```python
from build123d import *

# Parameters (mm, degrees)
SKETCH_1_R      = 1.4
SKETCH_1_W      = 12.8
SKETCH_1_H      = 6
SKETCH_1_W_2    = 15
SKETCH_1_W_3    = 6
SKETCH_1_H_2    = 10
EXTRUDE_1_DEPTH = 6


with BuildPart() as part:
    # Эскиз1 → Бобышка-Вытянуть1 (new body)
    with BuildSketch(Plane.XY):
        with BuildLine():
            Line((96.920798757, 2), (96.920798757, 25))
            Line((96.920798757, 25), (96.920798757, 33))
            ThreePointArc((96.920798757, 33), (98.385264851, 36.535533906), (101.920798757, 38))
            Line((101.920798757, 38), (149.389201243, 38))
            Line((149.389201243, 38), (149.389201243, 30))
            Line((149.389201243, 30), (149.389201243, 20.709265489))
            Line((149.389201243, 20.709265489), (143.389201243, 20.709265489))
            Line((143.389201243, 20.709265489), (143.389201243, 10.709265489))
            Line((143.389201243, 10.709265489), (149.389201243, 10.709265489))
            Line((149.389201243, 10.709265489), (149.389201243, -4.290734511))
            Line((149.389201243, -4.290734511), (143.389201243, -4.290734511))
            Line((143.389201243, -4.290734511), (143.389201243, -14.290734511))
            Line((143.389201243, -14.290734511), (149.389201243, -14.290734511))
            Line((149.389201243, -14.290734511), (149.389201243, -30))
            Line((149.389201243, -30), (-144.389201243, -30))
            Line((-144.389201243, -30), (-149.389201243, -25))
            Line((-149.389201243, -25), (-149.389201243, -13))
            Line((-149.389201243, -13), (81.920798757, -13))
            ThreePointArc((81.920798757, -13), (92.527400475, -8.606601718), (96.920798757, 2))
        make_face()
        with Locations((104.970798757, -19)):
            Circle(SKETCH_1_R, mode=Mode.SUBTRACT)
        with Locations((104.970798757, 25)):
            Circle(SKETCH_1_R, mode=Mode.SUBTRACT)
        with Locations((111.920798757, 3.209265489)):
            Circle(SKETCH_1_R, mode=Mode.SUBTRACT)
        with Locations((146.389201243, 3.209265489)):
            Circle(SKETCH_1_R, mode=Mode.SUBTRACT)
        with Locations((-128.98858016, -19)):
            Rectangle(SKETCH_1_W, SKETCH_1_H, mode=Mode.SUBTRACT)
        with Locations((-28.18858016, -19)):
            Rectangle(SKETCH_1_W, SKETCH_1_H, mode=Mode.SUBTRACT)
        with Locations((62.61141984, -19)):
            Rectangle(SKETCH_1_W, SKETCH_1_H, mode=Mode.SUBTRACT)
        with Locations((129.420798757, -19)):
            Rectangle(SKETCH_1_W_2, SKETCH_1_H, mode=Mode.SUBTRACT)
        with Locations((111.920798757, 15.709265489)):
            Rectangle(SKETCH_1_W_3, SKETCH_1_H_2, mode=Mode.SUBTRACT)
        with Locations((111.920798757, -9.290734511)):
            Rectangle(SKETCH_1_W_3, SKETCH_1_H_2, mode=Mode.SUBTRACT)
        with Locations((129.155798757, 33)):
            Rectangle(SKETCH_1_W_2, SKETCH_1_H, mode=Mode.SUBTRACT)
    extrude(amount=EXTRUDE_1_DEPTH)


solid = part.part
```
The model under review builds one solid part; all positions refer to its coordinate system, in mm. A direction names the side the tool comes from. Coordinates: 2 decimals unless noted, no trailing zeros. Write each loop counter-clockwise with the first axis right and the second up, starting at its lowest first coordinate (ties: lowest second). Pieces come first, ordered by that corner, then holes.
1) We need section B-B on x = -102. State the section outline as (y, z) points, then the cut area to 3 significant figures.
2) To check wall thickness, follow probe 1 along X at (y, z) = (-17, 2); probe 2 along Y at (x, z) = (135, 5.8); probe 3 along Y at (x, z) = (-128, 2.7). State the ranges of each line that lie inside material, in increasing order.
3) The part is to be moulded in two halves that separate along X. For faces 1 (the face through (-129, -22, 3)), 2 (the face through (149.389, 3, 3)), 3 (the face through (96.921, 17, 3)), say which applies: pulls with the +X half, pulls with the -X half, needs draft (parallel to the pull), parting line crosses it, or undercut.
4) We need section C-C on z = 2. Count the separate pieces of the cut face and the enclosed holes in it, then the cut area to 3 significant figures.
5) We need section A-A on y = -8.5. State the section outline as (x, z) points.
6) Clearance check with flat-ended pins moving along their axes: pin 1 Ø4.5 at (x, y) = (146.39, 3.21) entering from +Z; pin 2 Ø1.8 at (y, z) = (-7.5, 4) entering from +X; pin 3 Ø1.8 at (y, z) = (17, 4) entering from -X; pin 4 Ø3 at (x, z) = (-126.5, 4) entering from +Y. State where each tip first meets the part, or that it passes through.
7) Machinability: for faces 4 (the face through (146, 10.709, 3)), 5 (the face through (63, -22, 3)), 6 (the face through (-35, -13, 3)), which of the approach directions +Z, -Z, +X, -X, +Y, -Y give a long, thin tool a straight path to every point of the face, cutting with its end or side? Answer none if there is none.
Answer list:
1. outline: (-30, 0) - (-13, 0) - (-13, 6) - (-30, 6) - close
1. area: 102 mm2
2. probe 1: x = -149.39 to -135.39, -122.59 to -34.59, -21.79 to 56.21, 69.01 to 121.92, 136.92 to 149.39
2. probe 2: y = -30 to -22, -16 to 30, 36 to 38
2. probe 3: y = -30 to -22, -16 to -13
3. face 1: undercut
3. face 2: pulls with the +X half
3. face 3: pulls with the -X half
4. separate pieces: 1
4. enclosed holes: 11
4. area: 7,110 mm2
5. outline: (92.63, 0) - (108.92, 0) - (108.92, 6) - (92.63, 6) - close; (114.92, 0) - (143.39, 0) - (143.39, 6) - (114.92, 6) - close
6. pin 1: stops at z = 6
6. pin 2: stops at x = 143.39
6. pin 3: stops at x = 96.92
6. pin 4: stops at y = -13
7. face 4: +Z, -Z, +X
7. face 5: +Z, -Z
7. face 6: +Z, -Z, -X, +Y
